Could you check a few things on this drawing? It's one solid part, dimensions in mm from its lowest x, y, z. A direction names the side the tool comes from. Coordinates: 2 decimals unless noted, no trailing zeros. Order: outer loops, then holes, each group sorted by start corner. A loop starts at its lowest first (then second) coordinate and runs counter-clockwise, first axis right, second up. Notation, with made-up numbers: (29, 60.25) - (68, 60.25) arc R13 cw to (68, 84.25) - close; hole circle Ø8 at (35.5, -26.75). An arc over 180 degrees is marked (long way). Answer in a Markdown table with one row per item. Add a question column.
Item 1: I want a section at B-B (x = 5.5). Please give me the cut outline in (y, z).
Item 2: I want a section at D-D (z = 13). Please give me the cut outline in (x, y).
Item 3: On a 3-axis mill with a long thin cutter (end or side, diameter ignored), from which of +Z, -Z, +X, -X, +Y, -Y can I reach the whole of each face in a straight line? I mean the marked faces 1, 2, 3 and 4. Say none if no direction works.
Item 4: Thinking about a two-plate mould opening in Y: for the marked faces 5, 6 and 7, which applies, +Y half, -Y half, draft (parallel to the pull), parting line (faces both ways), or undercut?
Item 5: If I drill on line 1 along Y through (x, z) = (5.5, 7.75); line 2 along Y through (x, z) = (8.5, 4.25); line 3 along Y through (x, z) = (18.25, 9.5), over which ranges is the centre line in solid material (lowest first)? Write a range as from..to.
Item 6: I want a section at C-C (y = 18.5). Please give me the cut outline in (x, z), plus the area to 3 significant figures.
Item 7: I want a section at A-A (x = 9.5). Please give me the cut outline in (y, z).
Item 8: Will these pins go through, and if not, where does the flat tip stop? pin 1 Ø2 at (y, z) = (16.5, 12.5) entering from -X; pin 2 Ø1.5 at (x, y) = (9, 21.5) entering from +Z; pin 3 Ø3 at (x, y) = (12, 22.5) entering from -Z.
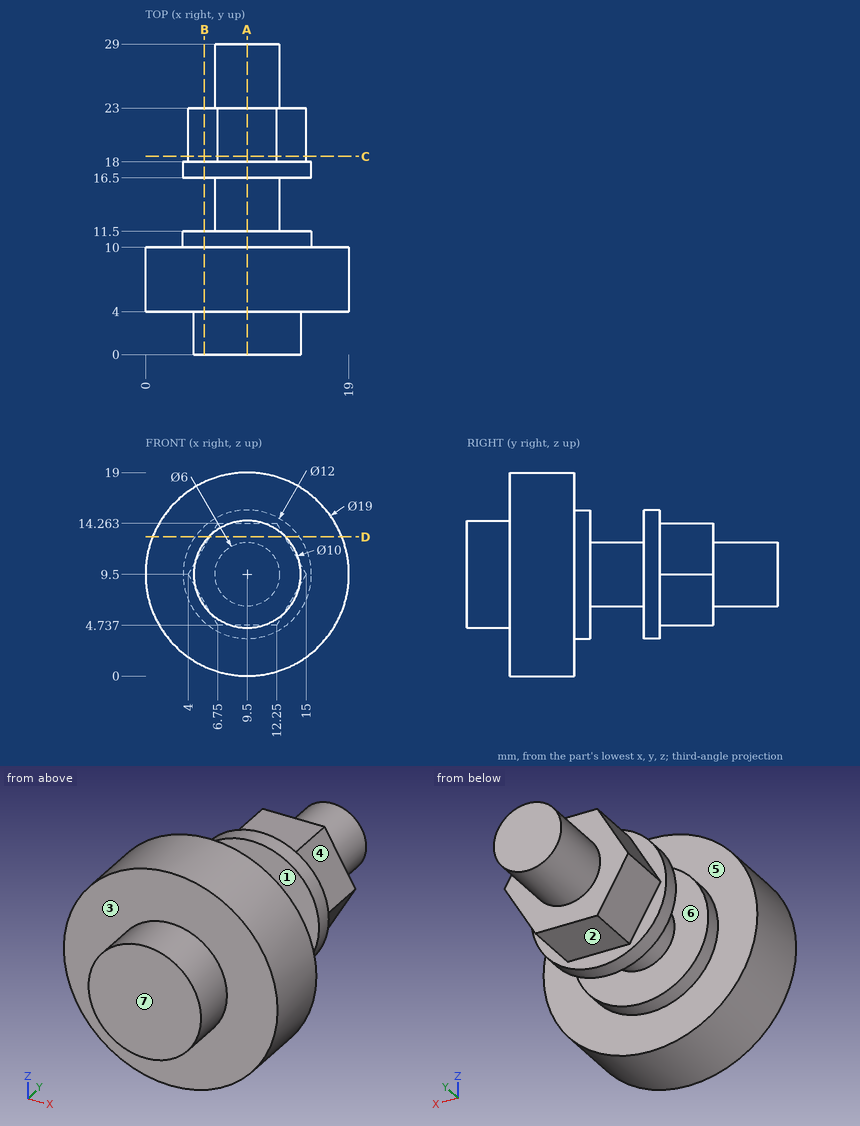
Values follow:
| question | item | result |
|---|---|---|
| 1 | outline | (0, 6.5) - (4, 6.5) - (4, 0.88) - (10, 0.88) - (10, 5.03) - (11.5, 5.03) - (11.5, 13.97) - (10, 13.97) - (10, 18.12) - (4, 18.12) - (4, 12.5) - (0, 12.5) - close; (16.5, 5.03) - (18, 5.03) - (18, 6.9) - (23, 6.9) - (23, 12.1) - (18, 12.1) - (18, 13.97) - (16.5, 13.97) - close |
| 2 | outline | (0.67, 4) - (5.93, 4) - (5.93, 0) - (13.07, 0) - (13.07, 4) - (18.33, 4) - (18.33, 10) - (14.37, 10) - (14.37, 11.5) - (4.63, 11.5) - (4.63, 10) - (0.67, 10) - close; (4.63, 16.5) - (14.37, 16.5) - (14.37, 18) - (12.98, 18) - (12.98, 23) - (6.02, 23) - (6.02, 18) - (4.63, 18) - close |
| 3 | face 1 | none |
| 3 | face 2 | -Z, +X, -X, +Y |
| 3 | face 3 | -Y |
| 3 | face 4 | +Z, +X, +Y |
| 4 | face 5 | +Y half |
| 4 | face 6 | undercut |
| 4 | face 7 | -Y half |
| 5 | line 1 | y = 0..11.5, 16.5..23 |
| 5 | line 2 | y = 4..11.5, 16.5..18 |
| 5 | line 3 | y = 4..10 |
| 6 | outline | (4, 9.5) - (6.75, 4.74) - (12.25, 4.74) - (15, 9.5) - (12.25, 14.26) - (6.75, 14.26) - close |
| 6 | area | 78.6 mm^2 |
| 7 | outline | (0, 4.5) - (4, 4.5) - (4, 0) - (10, 0) - (10, 3.5) - (11.5, 3.5) - (11.5, 6.5) - (16.5, 6.5) - (16.5, 3.5) - (18, 3.5) - (18, 4.74) - (23, 4.74) - (23, 6.5) - (29, 6.5) - (29, 12.5) - (23, 12.5) - (23, 14.26) - (18, 14.26) - (18, 15.5) - (16.5, 15.5) - (16.5, 12.5) - (11.5, 12.5) - (11.5, 15.5) - (10, 15.5) - (10, 19) - (4, 19) - (4, 14.5) - (0, 14.5) - close |
| 8 | pin 1 | stops at x = 3.84 |
| 8 | pin 2 | stops at z = 14.26 |
| 8 | pin 3 | stops at z = 4.74 |
